Autodesk Inventor part; units mm, degrees
ref_plane "YZ Plane" through (0, 0, 0) normal (1, 0, 0) x (0, 1, 0)
ref_plane "XZ Plane" through (0, 0, 0) normal (0, 1, 0) x (-1, 0, 0)
ref_plane "XY Plane" through (0, 0, 0) normal (0, 0, 1) x (1, 0, 0)
sketch "Sketch2" plane through (0, 0, 0) normal (0, 1, 0) x (-1, 0, 0)
  line L0 (457.2, 228.6) -> (-457.2, 228.6)
  line L1 (-457.2, 228.6) -> (-457.2, -228.6)
  line L2 (-457.2, -228.6) -> (457.2, -228.6)
  line L3 (457.2, -228.6) -> (457.2, 228.6)
  line L4 (457.2, 228.6) -> (-457.2, -228.6) construction
  line L5 (-457.2, 228.6) -> (457.2, -228.6) construction
  line L6 (454.025, 225.425) -> (-454.025, 225.425)
  line L7 (-454.025, 225.425) -> (-454.025, -225.425)
  line L8 (-454.025, -225.425) -> (454.025, -225.425)
  line L9 (454.025, -225.425) -> (454.025, 225.425)
  line L10 (454.025, 225.425) -> (-454.025, -225.425) construction
  line L11 (-454.025, 225.425) -> (454.025, -225.425) construction
  point P0 (0, 0)
  dimension "d0" = 914.4
  dimension "d1" = 457.2
  dimension "d2" = 3.175
  dimension "d3" = 3.175
extrude "Extrusion1" add sketch "Sketch2" along normal blind 304.8
extrude "Extrusion2" add sketch "Sketch2" along normal blind 12.7 contours L3 L2 L1 L0 | L9 L8 L7 L6
properties part number "Tank" material "Glass"
Input: part model. Units: mm. Frame: model coordinates. A direction names the side the tool comes from. Give positions to 0.01 mm unless a question says otherwise; leave off trailing zeros. Order: outer loops, then holes, each group sorted by start corner. A loop starts at its lowest first (then second) coordinate and runs counter-clockwise, first axis right, second up. Notation, with made-up numbers: M 20.25,-7 L 43.25,-7 A18 ccw 43.25,20 Z; hole C -15,-38.5 d11. An arc over 180 degrees is marked long. Return JSON: item names as keys, results as strings.
Item 1: Cut plane B-B (z = -192.5). Return loops of the section in (x, y) (3 decimals).
Solutions:
{"outline": "M -457.2,0 L 457.2,0 L 457.2,304.8 L 454.025,304.8 L 454.025,12.7 L -454.025,12.7 L -454.025,304.8 L -457.2,304.8 Z"}
Item 2: Access query for faces 4 (the flat face through (-454.025, 157, -3)), 5 (the flat face through (6, 150, -228.6)). Directions: +Z, -Z, +X, -X, +Y, -Y. A direction counts if a zero-diameter tool reaches every point of the face in a straight line with its end or side. Return the directions, or none.
Solutions:
{"face 4": "+Y", "face 5": "-Z, +X, -X, +Y, -Y"}
Item 3: Cut plane A-A (y = 225). Return loops of the section in (x, z) (3 decimals).
Solutions:
{"outline": "M -457.2,-228.6 L 457.2,-228.6 L 457.2,228.6 L -457.2,228.6 Z; hole M -454.025,-225.425 L 454.025,-225.425 L 454.025,225.425 L -454.025,225.425 Z"}
Item 4: Cut plane C-C (x = -253). Return loops of the section in (y, z) (3 decimals), then the cut area to 3 significant figures.
Solutions:
{"outline": "M 0,-228.6 L 304.8,-228.6 L 304.8,-225.425 L 12.7,-225.425 L 12.7,225.425 L 304.8,225.425 L 304.8,228.6 L 0,228.6 Z", "area": "7,660 mm^2"}
Item 5: Ray query, probe 1 along Z at (x, y) = (251.5, 284) (3 decimals); probe 2 along X at (y, z) = (65.5, -79) (3 decimals); probe 3 along Y at (x, z) = (352, 126). Return the intervals inside material, ascending.
Solutions:
{"probe 1": "-228.6 to -225.425, 225.425 to 228.6", "probe 2": "-457.2 to -454.025, 454.025 to 457.2", "probe 3": "0 to 12.7"}
Item 6: First-contact query: P1, Ø12, axis at x = -101.5, z = -130.5, coming from the +Y side. Flat tip, straight axial feed; report the tip coordinate or a pass-through.
Solutions:
{"P1": "y = 12.7"}
Item 7: Pull-direction query (X, two-part tool) for faces 1 (the flat face through (6, 157, -225.425)), 2 (the flat face through (-457.2, 150, -3)), 3 (the flat face through (6, 0, 3)); classes: +X half, -X half, draft (parallel to the pull), parting line (faces both ways), or undercut.
Solutions:
{"face 1": "undercut", "face 2": "-X half", "face 3": "draft"}
